```python
from build123d import *

# Parameters (mm, degrees)
EXTRUDE_1_DEPTH     = 150
SKETCH_3_R          = 30
EXTRUDE_2_DEPTH     = 75
SKETCH_4_R          = 50
CUT_EXTRUDE_1_DEPTH = 100


with BuildPart() as part:
    # 草图1 → 凸台-拉伸1 (new body)
    with BuildSketch(Plane.XY):
        Polygon((-100, 0), (100, 0), (100, 240), (188.822856765, 240), (150, 384.888873943), (-150, 384.888873943), (-188.822856765, 240), (-100, 240), align=None)
    extrude(amount=EXTRUDE_1_DEPTH)

    # 草图3 → 凸台-拉伸2 (add)
    with BuildSketch(Plane(origin=(236.17412377, 63.282665737, 0), x_dir=(0, 0, -1), z_dir=(0.9659258262890672, 0.2588190451025252, 0))):
        with Locations(Location((-75, 257.951246828, 0), (0, 0, 90))):
            Circle(SKETCH_3_R)
    extrude_2 = extrude(amount=EXTRUDE_2_DEPTH)

    # 镜向1: 凸台-拉伸2 across plane
    add(extrude_2.mirror(Plane.ZY))

    # 草图4 → 切除-拉伸1 (cut)
    with BuildSketch(Plane.XZ):
        with Locations(Location((0, 75, 0), (0, 0, 270))):
            Circle(SKETCH_4_R)
    extrude(amount=-CUT_EXTRUDE_1_DEPTH, mode=Mode.SUBTRACT)


solid = part.part
```
Check sheet for the modelled part. Datum: model origin and axes. Units: mm. A direction names the side the tool comes from. Coordinates: 2 decimals unless noted, no trailing zeros. Loops run counter-clockwise (first coordinate to the right, second up) from the corner with the lowest first, then second, coordinate; pieces in that order, holes last. Notation, with made-up numbers: M 52.25,-20.75 L 108.25,-20.75 A21 cw 108.25,4.25 Z; hole C 1.25,-23.5 d6. An arc over 180 degrees is marked long. Answer as a JSON object with one key per item and string values.
1. Release check for a two-part mould opening along Z. For faces 1 (the cylindrical face through (33.792, 49.3, 111.852)), 2 (the flat face through (-145, 240, 74)), 3 (the cylindrical face through (201, 337.6, 100.3)) record: pulls with the +Z half, pulls with the -Z half, needs draft (parallel to the pull), parting line crosses it, or undercut.
Outcome:
{"face 1": "undercut", "face 2": "needs draft", "face 3": "parting line crosses it"}
2. Sectioned sample at B-B on z = 14. Record the cut outline in (x, y).
Outcome:
{"outline": "M -188.82,240 L -100,240 L -100,0 L 100,0 L 100,240 L 188.82,240 L 150,384.89 L -150,384.89 Z"}
3. Scan lines: L1, parallel to X at y = 31, z = 75; L2, parallel to X at y = 160.5, z = 35.5; L3, parallel to X at y = 56, z = 87. Record each from-to range of solid material in increasing order. Write a range as from..to.
Outcome:
{"L1": "-100..-50, 50..100", "L2": "-100..100", "L3": "-100..-48.54, 48.54..100"}
4. Sectioned sample at A-A on x = 0. Record the cut outline in (y, z).
Outcome:
{"outline": "M 0,0 L 384.89,0 L 384.89,150 L 0,150 L 0,125 L 100,125 L 100,25 L 0,25 Z"}
5. Sectioned sample at C-C on y = 204. Record the cut outline in (x, z), and give its area (3 significant figures).
Outcome:
{"outline": "M -100,0 L 100,0 L 100,150 L -100,150 Z", "area": "30,000 mm²"}
6. Access from +Z, -Z, +X, -X, +Y, -Y to the whole of each face (thin tool, end or side, straight path). Record for faces 4 (the flat face through (-100, 122, 74)), 5 (the flat face through (1, 100, 76)), 6 (the flat face through (144, 240, 74)).
Outcome:
{"face 4": "+Z, -Z, -X, -Y", "face 5": "-Y", "face 6": "+Z, -Z, +X, -Y"}
7. Sectioned sample at D-D on z = 52.5. Record the cut outline in (x, y).
Outcome:
{"outline": "M -246.99,312.69 L -174.55,293.28 L -188.82,240 L -100,240 L -100,0 L -44.65,0 L -44.65,100 L 44.65,100 L 44.65,0 L 100,0 L 100,240 L 188.82,240 L 174.55,293.28 L 246.99,312.69 L 236.72,351.02 L 164.28,331.61 L 150,384.89 L -150,384.89 L -164.28,331.61 L -236.72,351.02 Z"}
8. Depth check by flat-ended pin: P1, Ø12, axis at x = -166.5, y = 293.5, coming from the -Z side; P2, Ø10, axis at y = 169, z = 118, coming from the +X side; P3, Ø2, axis at y = 113.5, z = 95, coming from the -X side. Enter the tip coordinate at first touch or a pass-through.
Outcome:
{"P1": "z = 0", "P2": "x = 100", "P3": "x = -100"}
